Part model, mm, in its own coordinate system. A direction names the side the tool comes from. Coordinates: 2 decimals unless noted, no trailing zeros. Write each loop counter-clockwise with the first axis right and the second up, starting at its lowest first coordinate (ties: lowest second). Pieces come first, ordered by that corner, then holes. Notation, with made-up numbers: M -38.5,11 L -24.5,11 A9 ccw -24.5,17 Z; hole C 1.25,37.5 d3. An arc over 180 degrees is marked long. Use a Markdown table: item, result. Add a question column.
Q1. Tool access for faces 1 (the cylindrical face through (-6.888, -47.587, -9.105)), 2 (the cylindrical face through (-22.463, -107.896, -16.152)), 3 (the flat face through (3, -56, -19.282)): list every direction of +Z, -Z, +X, -X, +Y, -Y with a clear straight run to the whole face (end or side of a thin tool).
Q2. Wall check: L1, parallel to X at y = -101.6, z = -14.75; L2, parallel to Y at x = -23, z = -14.75; L3, parallel to Y at x = 32, z = -15.5. Give the ranges that are in metal, low to high. Write a range as from..to.
Q3. Slice it at A-A on y = -50.8. Write the cut outline in (x, z).
Q4. Pin check, flat tips, straight feed: pin 1 Ø6.5 at (x, y) = (32, -13.5) entering from -Z; pin 2 Ø10 at (x, y) = (-19.5, -102.5) entering from -Z; pin 3 Ø2.5 at (x, y) = (14.5, -49.5) entering from +Z. Stop position of each tip, or through.
Q5. Slice it at C-C on x = 25. Write the cut outline in (y, z).
Q6. Slice it at B-B on z = -14.5. Write the cut outline in (x, y), then the cut area to 3 significant figures.
Q7. Mould opens along Y. For faces 4 (the flat face through (-34.336, -56, -14)), 5 (the flat face through (3, 0, -13)), 6 (the flat face through (3, -114.3, -13)), 7 (the cylindrical face through (13.656, -48.225, -9.105)) say: released by +Y, released by -Y, zero draft, split by the parting line, or undercut.
from build123d import *

# Parameters (mm, degrees)
F0_W     = 76.2
F0_H     = 11.43
F1_DEPTH = 114.3
F2_R     = 6.35
F3_DEPTH = 6.35
F4_R     = 3.81
F5_DEPTH = 2.54


with BuildPart() as f1:
    # F0 (on Front) → F1 (new body)
    with BuildSketch(Plane.XZ):
        with Locations((3.763746, -13.567377)):
            Rectangle(F0_W, F0_H)
    extrude(amount=F1_DEPTH)

    # F2 (on face) → F3 (cut)
    with BuildSketch(Plane(origin=(0, 0, -19.282377), x_dir=(1, 0, 0), z_dir=(0, 0, -1))):
        with Locations((-21.636254, 101.6)):
            Circle(F2_R)
        with Locations((29.163746, 101.6)):
            Circle(F2_R)
        with Locations((29.163746, 12.7)):
            Circle(F2_R)
        with Locations((-21.636254, 12.7)):
            Circle(F2_R)
    extrude(amount=-F3_DEPTH, mode=Mode.SUBTRACT)

    # F4 (on face) → F5 (cut)
    with BuildSketch(Plane.XY.offset(-7.852377)):
        with Locations((16.463746, -50.8)):
            Circle(F4_R)
        with Locations((-8.936254, -50.8)):
            Circle(F4_R)
    extrude(amount=-F5_DEPTH, mode=Mode.SUBTRACT)


solid = f1.part
Recorded:
| question | item | result |
|---|---|---|
| 1 | face 1 | +Z |
| 1 | face 2 | -Z |
| 1 | face 3 | -Z, +X, -X, +Y, -Y |
| 2 | L1 | -34.34..-27.99, -15.29..22.81, 35.51..41.86 |
| 2 | L2 | -114.3..-107.8, -95.4..-18.9, -6.5..0 |
| 2 | L3 | -114.3..-107.28, -95.92..-18.38, -7.02..0 |
| 3 | outline | M -34.34,-19.28 L 41.86,-19.28 L 41.86,-7.85 L 20.27,-7.85 L 20.27,-10.39 L 12.65,-10.39 L 12.65,-7.85 L -5.13,-7.85 L -5.13,-10.39 L -12.75,-10.39 L -12.75,-7.85 L -34.34,-7.85 Z |
| 4 | pin 1 | z = -12.93 |
| 4 | pin 2 | z = -19.28 |
| 4 | pin 3 | z = -10.39 |
| 5 | outline | M -114.3,-19.28 L -106.39,-19.28 L -106.39,-12.93 L -96.81,-12.93 L -96.81,-19.28 L -17.49,-19.28 L -17.49,-12.93 L -7.91,-12.93 L -7.91,-19.28 L 0,-19.28 L 0,-7.85 L -114.3,-7.85 Z |
| 6 | outline | M -34.34,-114.3 L 41.86,-114.3 L 41.86,0 L -34.34,0 Z; hole C -21.64,-101.6 d12.7; hole C -21.64,-12.7 d12.7; hole C 29.16,-101.6 d12.7; hole C 29.16,-12.7 d12.7 |
| 6 | area | 8,200 mm² |
| 7 | face 4 | zero draft |
| 7 | face 5 | released by +Y |
| 7 | face 6 | released by -Y |
| 7 | face 7 | undercut |
